Autodesk Inventor part; units mm, degrees
ref_plane "YZ Plane" through (0, 0, 0) normal (1, 0, 0) x (0, 1, 0)
ref_plane "XZ Plane" through (0, 0, 0) normal (0, 1, 0) x (-1, 0, 0)
ref_plane "XY Plane" through (0, 0, 0) normal (0, 0, 1) x (1, 0, 0)
sketch "스케치1" plane through (0, 0, 0) normal (0, 1, 0) x (-1, 0, 0)
  line L0 (-3.5031, -21.0217) -> (-3.5031, -19.0217)
  line L1 (-2.5031, -19.0217) -> (-2.5031, -16.0217)
  line L2 (-2.0031, -16.5217) -> (-0.0031, -16.5217)
  line L3 (-12.5031, -19.0217) -> (-12.5031, -21.0217)
  line L4 (-13.5031, -16.0217) -> (-13.5031, -19.0217)
  line L5 (-13.5031, -19.0217) -> (-2.5031, -19.0217)
  line L6 (-2.5031, -16.0217) -> (-13.5031, -16.0217)
  line L7 (-14.0031, -19.0217) -> (-2.0031, -19.0217)
  line L8 (-16.0031, -16.5217) -> (-14.0031, -16.5217)
  line L9 (-0.0031, -21.0217) -> (-16.0031, -21.0217)
  circle A0 centre (-8.0031, -10.5217) radius 5
  line L10 (-0.0031, -21.0217) -> (-0.0031, -0.0217)
  line L11 (-16.0031, -21.0217) -> (-16.0031, -0.0217)
  circle A1 centre (-8.0031, -10.5217) radius 7
  line L12 (-14.0031, -2.0217) -> (-14.0031, -19.0217)
  line L13 (-2.0031, -19.0217) -> (-2.0031, -2.0217)
  line L14 (-2.0031, -4.5217) -> (-0.0031, -4.5217)
  line L15 (-3.5031, -2.0217) -> (-3.5031, -0.0217)
  line L16 (-12.5031, -2.0217) -> (-12.5031, -0.0217)
  line L17 (-14.0031, -4.5217) -> (-16.0031, -4.5217)
  line L18 (-2.0031, -2.0217) -> (-14.0031, -2.0217)
  line L19 (-16.0031, -0.0217) -> (-0.0031, -0.0217)
  circle A2 centre (-8.0031, -10.5217) radius 2.25
  point P0 (0, 0)
  point P1 (-2.0031, -6.9161)
  point P2 (-2.0031, -14.1272)
  point P3 (-14.0031, -14.1272)
  point P4 (-14.0031, -6.9161)
  dimension "d0" = 21
  dimension "d1" = 4.5
  dimension "d19" = 17
  dimension "d20" = 12
  dimension "d21" = 10
extrude "돌출2" add sketch "스케치1" against normal blind 12 contours L9 L3 L5 L0 | L0 L5 L7 L13 L2 L10 L9 | L9 L11 L8 L12 L7 L5 L3 | L2 L13 A1 L14 L10 | L14 L13 L18 L15 L19 L10 | L11 L17 L12 A1 L8 | L11 L19 L16 L18 L12 L17 | L15 L18 L16 L19
extrude "돌출3" add sketch "스케치1" along normal blind 5 contours L9 L3 L5 L0 | L0 L5 L7 L13 L2 L10 L9 | L5 L4 L6 A1 L1 | L9 L11 L8 L12 L7 L5 L3 | L1 L6 A1 L13 L7 | L2 L13 A1 L14 L10 | L7 L12 A1 L6 L4 | L14 L13 L18 L15 L19 L10 | L11 L17 L12 A1 L8 | A1 L6 | L6 A1 L12 L13 | L13 A1 | L13 A1 L12 L18 | L11 L19 L16 L18 L12 L17 | L15 L18 L16 L19 | A1 L12 | A0 | A2
extrude "돌출4" cut sketch "스케치1" along normal blind 13 contours A2
sketch "스케치2" plane through (0, 5, 0) normal (0, 1, 0) x (1, 0, 0)
  point P0 (0, 0)
  point P1 (8.0031, 10.5217)
sketch "스케치3" plane through (0, 5, 0) normal (0, 1, 0) x (1, 0, 0)
  circle A0 centre (8.0031, 10.5217) radius 2.25
  circle A1 centre (8.0031, 10.5217) radius 5
  point P0 (0, 0)
  dimension "d10" = 10
fillet "모깎기1" radius 3 4 edges at (16.0031, -3.5, -21.0217) (0.0031, -3.5, -21.0217) (16.0031, -3.5, -0.0217) (0.0031, -3.5, -0.0217)
chamfer "모따기1" distance 5 angle 45 1 edges at (10.2531, 5, -10.5217) measured on face at (1.9198, 5, -10.5217)
properties part number "센서부 90"
Verification items for the finished model (mm, model axes). A direction names the side the tool comes from. Give positions to 0.01 mm unless a question says otherwise; leave off trailing zeros. Loops run counter-clockwise (first coordinate to the right, second up) from the corner with the lowest first, then second, coordinate; pieces in that order, holes last.
1. Cross-section at C-C on y = 3.5. Record the cut outline in (x, z).
Derived:
outline: (0, -18.02) arc R3 ccw to (3, -21.02) - (13, -21.02) arc R3 ccw to (16, -18.02) - (16, -3.02) arc R3 ccw to (13, -0.02) - (3, -0.02) arc R3 ccw to (0, -3.02) - close; hole circle Ø11.5 at (8, -10.52)
2. Release check for a two-part mould opening along X. For faces 1 (the flat face through (8, -6, -2.022)), 2 (the flat face through (14.003, -6, -4)), 3 (the cylindrical face through (15.101, -3.619, -20.166)), 4 (the cylindrical face through (0.86, -3.38, -0.92)) record: +X half, -X half, draft (parallel to the pull), parting line (faces both ways), or undercut.
Derived:
face 1: undercut
face 2: undercut
face 3: +X half
face 4: -X half
3. Cross-section at A-A on y = -0.75. Record the cut outline in (x, z).
Derived:
outline: (0, -18.02) arc R3 ccw to (3, -21.02) - (13, -21.02) arc R3 ccw to (16, -18.02) - (16, -3.02) arc R3 ccw to (13, -0.02) - (3, -0.02) arc R3 ccw to (0, -3.02) - close; hole (2, -19.02) - (14, -19.02) - (14, -14.13) arc R7 ccw to (14, -6.92) - (14, -2.02) - (2, -2.02) - (2, -6.92) arc R7 ccw to (2, -14.13) - close
4. Cross-section at B-B on y = 1.5. Record the cut outline in (x, z), and give its area (3 significant figures).
Derived:
outline: (0, -18.02) arc R3 ccw to (3, -21.02) - (13, -21.02) arc R3 ccw to (16, -18.02) - (16, -3.02) arc R3 ccw to (13, -0.02) - (3, -0.02) arc R3 ccw to (0, -3.02) - close; hole circle Ø7.5 at (8, -10.52)
area: 284 mm2
5. Go/stop test with flat-tipped pins: P1, Ø2, axis at x = 8.5, z = -14, coming from the +Y side; P2, Ø6, axis at x = 8, z = -10.52, coming from the -Y side. Record where each tip stops, or that it passes through.
Derived:
P1: stops at y = 2.26
P2: stops at y = 0
6. Tool access check on faces 5 (the flat face through (15.2, -12, -10.4)), 6 (the cylindrical face through (15.003, -5.916, -10.469)). Record the directions out of +Z, -Z, +X, -X, +Y, -Y that give a thin tool (end or side, any length) a straight path to the whole face; none if there is none.
Derived:
face 5: +Z, -Z, +X, -X, -Y
face 6: -Y
7. Material ranges on probe 1 along X at (y, z) = (-7, -3); probe 2 along Z at (x, y) = (11.75, -10.75); probe 3 along Z at (x, y) = (2.5, -2.5), recorded low to high.
Derived:
probe 1: x = 0 to 2, 14 to 16
probe 2: z = -21.02 to -19.02, -2.02 to -0.02
probe 3: z = -20.98 to -19.02, -2.02 to -0.06
